from build123d import *

# Parameters (mm, degrees)
EXTRUDE_1_DEPTH     = 3
SKETCH_4_W          = 15
SKETCH_4_H          = 21
CUT_EXTRUDE_1_DEPTH = 3
SKETCH_5_R          = 1.55
CUT_EXTRUDE_2_DEPTH = 272.724124803
SKETCH_7_W          = 21
SKETCH_7_H          = 75
CUT_EXTRUDE_3_DEPTH = 272.724124803
SKETCH_8_R          = 2.1
CUT_EXTRUDE_4_DEPTH = 272.724124803
SKETCH_9_R          = 2.1
CUT_EXTRUDE_5_DEPTH = 272.724124803


with BuildPart() as part:
    # 草图1 → 凸台-拉伸1 (new body)
    with BuildSketch(Plane.XY):
        Polygon((0, 240), (0, 265), (60, 265), (60, 240), (60, 0), (0, 0), align=None)
    extrude(amount=EXTRUDE_1_DEPTH)

    # 草图4 → 切除-拉伸1 (cut)
    with BuildSketch(Plane(origin=(0, 0, 0), x_dir=(-1, 0, 0), z_dir=(0, 0, -1))):
        with Locations((-52.5, 17.5)):
            Rectangle(SKETCH_4_W, SKETCH_4_H)
        with Locations((-7.5, 17.5)):
            Rectangle(SKETCH_4_W, SKETCH_4_H)
        with Locations((-7.5, 197.5)):
            Rectangle(SKETCH_4_W, SKETCH_4_H)
        with Locations((-52.5, 197.5)):
            Rectangle(SKETCH_4_W, SKETCH_4_H)
    extrude(amount=-CUT_EXTRUDE_1_DEPTH, mode=Mode.SUBTRACT)

    # 草图5 → 切除-拉伸2 (cut, through all)
    with BuildSketch(Plane(origin=(0, 0, 0), x_dir=(-1, 0, 0), z_dir=(0, 0, -1))):
        with Locations((-45, 229.6)):
            Circle(SKETCH_5_R)
        with Locations((-45, 253.6)):
            Circle(SKETCH_5_R)
        with Locations((-15, 253.6)):
            Circle(SKETCH_5_R)
        with Locations((-15, 229.6)):
            Circle(SKETCH_5_R)
        with Locations((-57, 184.75)):
            Circle(SKETCH_5_R)
        with Locations((-3, 184.75)):
            Circle(SKETCH_5_R)
        with Locations((-3, 210.85)):
            Circle(SKETCH_5_R)
        with Locations((-57, 210.85)):
            Circle(SKETCH_5_R)
        with Locations((-57, 4.75)):
            Circle(SKETCH_5_R)
        with Locations((-3, 4.75)):
            Circle(SKETCH_5_R)
        with Locations((-3, 30.85)):
            Circle(SKETCH_5_R)
        with Locations((-57, 30.85)):
            Circle(SKETCH_5_R)
    extrude(amount=-CUT_EXTRUDE_2_DEPTH, mode=Mode.SUBTRACT)

    # 草图7 → 切除-拉伸3 (cut, through all)
    with BuildSketch(Plane(origin=(0, 0, 0), x_dir=(-1, 0, 0), z_dir=(0, 0, -1))):
        with Locations((-49.5, 77.5)):
            Rectangle(SKETCH_7_W, SKETCH_7_H)
    extrude(amount=-CUT_EXTRUDE_3_DEPTH, mode=Mode.SUBTRACT)

    # 草图8 → 切除-拉伸4 (cut, through all)
    with BuildSketch(Plane.XY.offset(3)):
        with Locations((31, 160.7)):
            Circle(SKETCH_8_R)
        with Locations((31, 124.7)):
            Circle(SKETCH_8_R)
    extrude(amount=-CUT_EXTRUDE_4_DEPTH, mode=Mode.SUBTRACT)

    # 草图9 → 切除-拉伸5 (cut, through all)
    with BuildSketch(Plane(origin=(0, 0, 0), x_dir=(-1, 0, 0), z_dir=(0, 0, -1))):
        with Locations((-17, 71.6)):
            Circle(SKETCH_9_R)
        with Locations((-33, 71.6)):
            Circle(SKETCH_9_R)
    extrude(amount=-CUT_EXTRUDE_5_DEPTH, mode=Mode.SUBTRACT)


solid = part.part
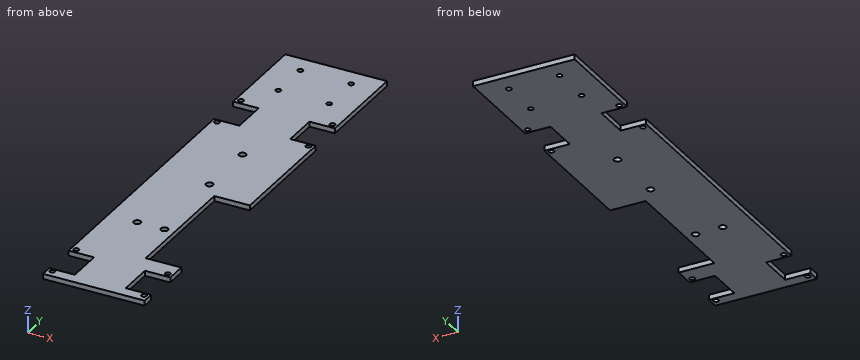
Input: part model. Units: mm. Frame: model coordinates. Give positions to 0.01 mm unless a question says otherwise; leave off trailing zeros. Write each loop counter-clockwise with the first axis right and the second up, starting at its lowest first coordinate (ties: lowest second). Pieces come first, ordered by that corner, then holes. Notation, with made-up numbers: M -16.5,49 L -12.5,49 A15 ccw -12.5,77 Z; hole C 53.25,37 d4. An arc over 180 degrees is marked long. Use one line per item in the form item = value.
1. First-contact query: P1, Ø0.9, axis at y = 201.5, z = 1, coming from the -X side; P2, Ø3, axis at x = 15, y = 253.6, coming from the +Z side. Flat tips, straight axial feed; report the tip coordinate or a pass-through.
Outcome:
P1 = 15
P2 = through
2. Cut plane A-A on z = 1.95. State how many separate pieces and enclosed holes the cut face has, and give its area (3 significant figures).
Outcome:
separate_pieces = 1
enclosed_holes = 16
area = 12,900 mm²
3. Cut plane B-B on y = 44. Return loops of the section in (x, z).
Outcome:
outline = M 0,0 L 39,0 L 39,3 L 0,3 Z
4. Ray query, L1, parallel to X at y = 184.75, z = 1.35; L2, parallel to Y at x = 48, z = 2.3; L3, parallel to Y at x = 6, z = 1.5. Return the intervals inside material, ascending.
Outcome:
L1 = 0 to 1.45, 4.55 to 55.45, 58.55 to 60
L2 = 0 to 7, 28 to 40, 115 to 187, 208 to 265
L3 = 0 to 7, 28 to 187, 208 to 265
